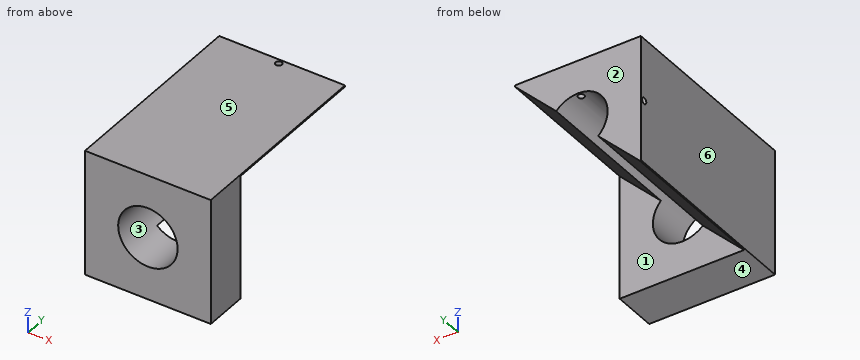
```python
from build123d import *

# Parameters (mm, degrees)
SKETCH1_W                             = 12.7
SKETCH1_H                             = 12.7
BOSS_EXTRUDE1_DEPTH                   = 20
SKETCH2_R                             = 3
CUT_EXTRUDE1_DEPTH                    = 27.880848201
CUT_EXTRUDE2_DEPTH                    = 15.6
F_72_0_025_DIAMETER_HOLE1_D           = 0.635
F_72_0_025_DIAMETER_HOLE1_ON_FACE_2_D = 0.635


with BuildPart() as part:
    # Sketch1 → Boss-Extrude1 (new body)
    with BuildSketch(Plane(origin=(0, 0, 0), x_dir=(1, 0, 0), z_dir=(0, 1, 0))):
        with Locations((6.35, 6.35)):
            Rectangle(SKETCH1_W, SKETCH1_H)
    extrude(amount=BOSS_EXTRUDE1_DEPTH)

    # Sketch2 → Cut-Extrude1 (cut, through all)
    with BuildSketch(Plane(origin=(0, 20, 0), x_dir=(1, 0, 0), z_dir=(0, 1, 0))):
        with Locations(Location((6.35, 6.35, 0), (0, 0, 270))):
            Circle(SKETCH2_R)
    extrude(amount=-CUT_EXTRUDE1_DEPTH, mode=Mode.SUBTRACT)

    # Sketch3 → Cut-Extrude2 (cut)
    with BuildSketch(Plane(origin=(0, 20, 0), x_dir=(1, 0, 0), z_dir=(0, 1, 0))):
        Polygon((12.7, 0.143684098), (0.143684098, 12.7), (12.7, 12.7), align=None)
    extrude(amount=-CUT_EXTRUDE2_DEPTH, mode=Mode.SUBTRACT)

    # #72 (0.025) Diameter Hole1 (through all)
    with Locations(Plane(origin=(6.35, 19.5, 0), x_dir=(1, 0, 0), z_dir=(0, 0, 1))):
        with Locations((0, 0)):
            Hole(F_72_0_025_DIAMETER_HOLE1_D / 2)

    # #72 (0.025) Diameter Hole1 on face 2 (through all)
    with Locations(Plane(origin=(0, 19.5, -6.35), x_dir=(0, 0, -1), z_dir=(-1, 0, 0))):
        with Locations((0, 0)):
            Hole(F_72_0_025_DIAMETER_HOLE1_ON_FACE_2_D / 2)


solid = part.part
```
Input: part model. Units: mm. Frame: model coordinates. Face numbers are marked on the shaded views. A direction names the side the tool comes from. Coordinates: 2 decimals unless noted, no trailing zeros. Write each loop counter-clockwise with the first axis right and the second up, starting at its lowest first coordinate (ties: lowest second). Pieces come first, ordered by that corner, then holes. Notation, with made-up numbers: (49.5, 61.5) - (107.5, 61.5) arc R13 ccw to (107.5, 83.5) - close; hole circle Ø9 at (4, 44.5). An arc over 180 degrees is marked (long way). Put each result on its own line as item: value. Start each with the question number.
1) Cut plane A-A (y = 19.5). Return the cut outline in (x, z), plus the area to 3 significant figures.
2) Cut plane B-B (x = 6.35). Return the cut outline in (y, z).
3) Mould query, pull axis Z, two halves, no side actions, for the marked faces 3, 4, 5 and 6. Classes: pulls with the +Z half, pulls with the -Z half, needs draft (parallel to the pull), parting line crosses it, or undercut.
4) Cut plane C-C (y = 3). Return the cut outline in (x, z), plus the area to 3 significant figures.
5) Reachability of the marked faces 1 and 2 from +Z, -Z, +X, -X, +Y, -Y: full face, straight path, thin tool, end or side. Return the list, or none.
6) Ray query, L1, parallel to Y at x = 6.35, z = -2.5; L2, parallel to Y at x = 10.75, z = -2.5; L3, parallel to X at y = 19.5, z = -2. Return the intervals inside material, ascending.
7) Contact query for flat-ended pins moving along their axis: pin 1 (5 mm diameter, centred on x = 6.35, z = -6.35, fed in from -Y); pin 2 (3 mm diameter, centred on y = 9.5, z = -11.5, fed in from -X); pin 3 (4 mm diameter, centred on y = 15, z = -9, fed in from +X). Output: stop coordinate, or through.
Resolved:
1. outline: (0, -12.7) - (0.14, -12.7) - (4.3, -8.54) arc R3 cw to (3.37, -6.67) - (0, -6.67) - close; (0, -6.03) - (3.37, -6.03) arc R3 cw to (6.03, -3.37) - (6.03, 0) - (0, 0) - close; (6.67, -3.37) arc R3 cw to (8.54, -4.3) - (12.7, -0.14) - (12.7, 0) - (6.67, 0) - close
1. area: 63.5 mm2
2. outline: (0, -12.7) - (4.4, -12.7) - (4.4, -9.35) - (0, -9.35) - close; (0, -3.35) - (19.18, -3.35) - (19.18, 0) - (0, 0) - close; (19.82, -3.35) - (20, -3.35) - (20, 0) - (19.82, 0) - close
3. face 3: undercut
3. face 4: pulls with the -Z half
3. face 5: pulls with the +Z half
3. face 6: needs draft
4. outline: (0, -12.7) - (12.7, -12.7) - (12.7, 0) - (0, 0) - close; hole circle Ø6 at (6.35, -6.35)
4. area: 133 mm2
5. face 1: -Z, +X, +Y
5. face 2: +Z, -Z, +X, -X, +Y
6. L1: y = 0 to 19.18, 19.82 to 20
6. L2: y = 0 to 4.4
6. L3: x = 0 to 6.03, 6.67 to 10.84
7. pin 1: passes through
7. pin 2: stops at x = 0
7. pin 3: stops at x = 4.3
